The model under review builds one solid part; all positions refer to its coordinate system, in mm. A direction names the side the tool comes from. Coordinates: 2 decimals unless noted, no trailing zeros. Order: outer loops, then holes, each group sorted by start corner. A loop starts at its lowest first (then second) coordinate and runs counter-clockwise, first axis right, second up. Notation, with made-up numbers: (14, -18) - (51, -18) arc R22 cw to (51, 7) - close; hole circle Ø6 at (2.25, -15.5). An arc over 180 degrees is marked (long way). Answer in a Markdown table with one row per item.
```python
from build123d import *

# Parameters (mm, degrees)
F1_DEPTH = 100
F2_R     = 11.25
F3_DEPTH = 25
F4_R     = 3.5
F5_DEPTH = 25


with BuildPart() as f1:
    # F0 (on Front) → F1 (new body)
    with BuildSketch(Plane.XZ):
        with BuildLine():
            Line((-93.888451, 0), (-106.888451, 0))
            Line((-106.888451, 0), (-106.888451, -2))
            Line((-106.888451, -2), (-93.888451, -2))
            ThreePointArc((-93.888451, -2), (-91.060024, -0.828427), (-89.888451, 2))
            Line((-89.888451, 2), (-89.888451, 94))
            ThreePointArc((-89.888451, 94), (-89.302665, 95.414214), (-87.888451, 96))
            Line((-87.888451, 96), (24.111549, 96))
            ThreePointArc((24.111549, 96), (25.525762, 95.414214), (26.111549, 94))
            Line((26.111549, 94), (26.111549, 2))
            ThreePointArc((26.111549, 2), (27.283121, -0.828427), (30.111549, -2))
            Line((30.111549, -2), (43.111549, -2))
            Line((43.111549, -2), (43.111549, 0))
            Line((43.111549, 0), (30.111549, 0))
            ThreePointArc((30.111549, 0), (28.697335, 0.585786), (28.111549, 2))
            Line((28.111549, 2), (28.111549, 94))
            ThreePointArc((28.111549, 94), (26.939976, 96.828427), (24.111549, 98))
            Line((24.111549, 98), (-87.888451, 98))
            ThreePointArc((-87.888451, 98), (-90.716879, 96.828427), (-91.888451, 94))
            Line((-91.888451, 94), (-91.888451, 2))
            ThreePointArc((-91.888451, 2), (-92.474238, 0.585786), (-93.888451, 0))
        make_face()
    extrude(amount=F1_DEPTH)

    # F2 (on face) → F3 (cut)
    with BuildSketch(Plane.XY.offset(98)):
        with Locations((-6.888451, -65)):
            Circle(F2_R)
    extrude(amount=-F3_DEPTH, mode=Mode.SUBTRACT)

    # F4 (on face) → F5 (cut)
    with BuildSketch(Plane(origin=(0, 0, -2), x_dir=(1, 0, 0), z_dir=(0, 0, -1))):
        with Locations((37.111549, 90)):
            Circle(F4_R)
        with Locations((37.111549, 10)):
            Circle(F4_R)
        with Locations((-100.888451, 10)):
            Circle(F4_R)
        with Locations((-100.888451, 90)):
            Circle(F4_R)
    extrude(amount=-F5_DEPTH, mode=Mode.SUBTRACT)


solid = f1.part
```
Item 1: We need section D-D, the plane x = -16. Write out the cut boundary in (y, z), then the cut area to 3 significant figures.
Check values:
| item | result |
|---|---|
| outline | (-100, 96) - (-71.6, 96) - (-71.6, 98) - (-100, 98) - close; (-58.4, 96) - (0, 96) - (0, 98) - (-58.4, 98) - close |
| area | 174 mm^2 |
Item 2: We need section B-B, the plane y = -65. Write out the cut boundary in (x, z).
Check values:
| item | result |
|---|---|
| outline | (-106.89, -2) - (-93.89, -2) arc R4 ccw to (-89.89, 2) - (-89.89, 94) arc R2 cw to (-87.89, 96) - (-18.14, 96) - (-18.14, 98) - (-87.89, 98) arc R4 ccw to (-91.89, 94) - (-91.89, 2) arc R2 cw to (-93.89, 0) - (-106.89, 0) - close; (4.36, 96) - (24.11, 96) arc R2 cw to (26.11, 94) - (26.11, 2) arc R4 ccw to (30.11, -2) - (43.11, -2) - (43.11, 0) - (30.11, 0) arc R2 cw to (28.11, 2) - (28.11, 94) arc R4 ccw to (24.11, 98) - (4.36, 98) - close |
Item 3: To check wall thickness, follow line 1 (X direction, y = -46, z = 58); line 2 (Z direction, x = -63, y = -12); line 3 (X direction, y = -10, z = -1). State the ranges of each line that lie inside material, in increasing order. Write a range as from..to.
Check values:
| item | result |
|---|---|
| line 1 | -91.89..-89.89, 26.11..28.11 |
| line 2 | 96..98 |
| line 3 | -106.89..-104.39, -97.39..-91.24, 27.47..33.61, 40.61..43.11 |
Item 4: We need section C-C, the plane y = -90. Write out the cut boundary in (x, z).
Check values:
| item | result |
|---|---|
| outline | (-106.89, -2) - (-104.39, -2) - (-104.39, 0) - (-106.89, 0) - close; (-97.39, -2) - (-93.89, -2) arc R4 ccw to (-89.89, 2) - (-89.89, 94) arc R2 cw to (-87.89, 96) - (24.11, 96) arc R2 cw to (26.11, 94) - (26.11, 2) arc R4 ccw to (30.11, -2) - (33.61, -2) - (33.61, 0) - (30.11, 0) arc R2 cw to (28.11, 2) - (28.11, 94) arc R4 ccw to (24.11, 98) - (-87.89, 98) arc R4 ccw to (-91.89, 94) - (-91.89, 2) arc R2 cw to (-93.89, 0) - (-97.39, 0) - close; (40.61, -2) - (43.11, -2) - (43.11, 0) - (40.61, 0) - close |
Item 5: We need section A-A, the plane z = 15. Write out the cut boundary in (x, y), then the cut area to 3 significant figures.
Check values:
| item | result |
|---|---|
| outline | (-91.89, -100) - (-89.89, -100) - (-89.89, 0) - (-91.89, 0) - close; (26.11, -100) - (28.11, -100) - (28.11, 0) - (26.11, 0) - close |
| area | 400 mm^2 |
Item 6: Tool access review of faces 4 (the face through (28.112, -49, 47)), 5 (the face through (-100, -49, 0)), 6 (the face through (34.334, -7.87, -1.014)), 7 (the face through (-33, -49, 96)): name each direction out of +Z, -Z, +X, -X, +Y, -Y from which nothing blocks a thin tool from reaching the whole face with its end or side.
Check values:
| item | result |
|---|---|
| face 4 | +Z, +X, +Y, -Y |
| face 5 | +Z, -X, +Y, -Y |
| face 6 | +Z, -Z |
| face 7 | -Z, +Y, -Y |
Item 7: Mouldability with a two-part tool opening along X and no side actions: class faces 1 (the face through (26.112, -49, 49)), 2 (the face through (37, -49, 0)), 3 (the face through (-91.888, -49, 49)) as +X half, -X half, draft (parallel to the pull), parting line (faces both ways), or undercut.
Check values:
| item | result |
|---|---|
| face 1 | undercut |
| face 2 | draft |
| face 3 | -X half |
Item 8: Clearance check with flat-ended pins moving along their axes: pin 1 Ø8 at (x, y) = (-75, -75) entering from -Z; pin 2 Ø10 at (y, z) = (-24, 28.5) entering from +X; pin 3 Ø4 at (x, y) = (-101.5, -51.5) entering from +Z. State where each tip first meets the part, or that it passes through.
Check values:
| item | result |
|---|---|
| pin 1 | z = 96 |
| pin 2 | x = 28.11 |
| pin 3 | z = 0 |
